Can you work these out from the model? Positions are in its coordinate system, mm. A direction names the side the tool comes from. Give positions to 0.01 mm unless a question says otherwise; leave off trailing zeros. Write each loop counter-clockwise with the first axis right and the second up, starting at its lowest first coordinate (ties: lowest second). Pieces come first, ordered by that corner, then holes. Notation, with made-up numbers: (21, -25.75) - (68, -25.75) arc R8 cw to (68, -18.75) - close; hole circle Ø2 at (-33.5, 26). An arc over 180 degrees is marked (long way). Return JSON: item names as keys, results as strings. Group by question number.
from build123d import *

# Parameters (mm, degrees)
SKETCH1_R           = 7.5
SKETCH1_R_2         = 2.3
BOSS_EXTRUDE1_DEPTH = 3.2
BOSS_EXTRUDE2_DEPTH = 2
CIRPATTERN1_COUNT   = 24


with BuildPart() as part:
    # Sketch1 → Boss-Extrude1 (new body)
    with BuildSketch(Plane(origin=(0, 0, 0), x_dir=(1, 0, 0), z_dir=(0, 1, 0))):
        with Locations(Location((0, 0, 0), (0, 0, 270))):
            Circle(SKETCH1_R)
        with Locations(Location((0, 0, 0), (0, 0, 270))):
            Circle(SKETCH1_R_2, mode=Mode.SUBTRACT)
    extrude(amount=BOSS_EXTRUDE1_DEPTH)

    # Sketch2 → Boss-Extrude2 (add)
    with BuildSketch(Plane.XZ):
        Polygon((9.114493261, 0.25), (9.114493261, -0.25), (7.314493261, -0.75), (7.314493261, 0.75), align=None)
    boss_extrude2 = extrude(amount=-BOSS_EXTRUDE2_DEPTH)

    # CirPattern1: Boss-Extrude2 ×24 about axis
    cirpattern1_axis = Axis((0, 0, 0), (0, 1, 0))
    for i in range(1, CIRPATTERN1_COUNT):
        add(boss_extrude2.rotate(cirpattern1_axis, i * 360 / CIRPATTERN1_COUNT))


solid = part.part
1) Imagine slicing it at C-C, the plane y = 2.3. Write out the boundary of the cut face in (x, z), and give its area (3 significant figures).
2) I need wall thicknesses on line 1 along X through (y, z) = (0.65, -7.25); line 2 along X through (y, z) = (1.6, 0); line 3 along X through (y, z) = (2.15, 0). Which ranges of each line are inside material? Lowest first, please.
3) Imagine slicing it at B-B, the plane x = 0. Write out the boundary of the cut face in (y, z), and give its area (3 significant figures).
4) Imagine slicing it at A-A, the plane z = 0. Write out the boundary of the cut face in (x, y).
5) Imagine slicing it at D-D, the plane x = 3.5. Write out the boundary of the cut face in (y, z).
6) Will these pins go through, and if not, where does the flat tip stop? pin 1 Ø0.9 at (x, z) = (6, -5.5) entering from +Y; pin 2 Ø1.5 at (x, y) = (-2, 2) entering from -Z; pin 3 Ø1.5 at (y, z) = (1, 6.5) entering from -X.
7) On a 3-axis mill with a long thin cutter (end or side, diameter ignored), from which of +Z, -Z, +X, -X, +Y, -Y can I reach the whole of each face in a straight line? I mean faces 1 (the face through (7.43, 0.99, 3.74)), 2 (the face through (2, 2, 8)), 3 (the face through (-6.207, 0.986, -5.534)), 4 (the face through (-8, 2, 2)). Say none if no direction works.
Resolved:
{
 "1": {"outline": "circle Ø15 at (0, 0); hole circle Ø4.6 at (0, 0)", "area": "160 mm^2"},
 "2": {"line 1": "-4.64 to -3.56, -2.61 to 2.61, 3.56 to 4.64", "line 2": "-9.11 to -2.3, 2.3 to 9.11", "line 3": "-7.5 to -2.3, 2.3 to 7.5"},
 "3": {"outline": "(0, -9.11) - (2, -9.11) - (2, -7.5) - (3.2, -7.5) - (3.2, -2.3) - (0, -2.3) - close; (0, 2.3) - (3.2, 2.3) - (3.2, 7.5) - (2, 7.5) - (2, 9.11) - (0, 9.11) - close", "area": "39.7 mm^2"},
 "4": {"outline": "(-9.11, 0) - (-2.3, 0) - (-2.3, 3.2) - (-7.5, 3.2) - (-7.5, 2) - (-9.11, 2) - close; (2.3, 0) - (9.11, 0) - (9.11, 2) - (7.5, 2) - (7.5, 3.2) - (2.3, 3.2) - close"},
 "5": {"outline": "(0, -7.19) - (2, -7.19) - (2, -6.63) - (3.2, -6.63) - (3.2, 6.63) - (2, 6.63) - (2, 7.19) - (0, 7.19) - close"},
 "6": {"pin 1": "y = 2", "pin 2": "z = -8.87", "pin 3": "x = -6.62"},
 "7": {"face 1": "+X, +Y, -Y", "face 2": "+Z, +X, +Y", "face 3": "-X, +Y, -Y", "face 4": "+Z, -X, +Y"}
}
